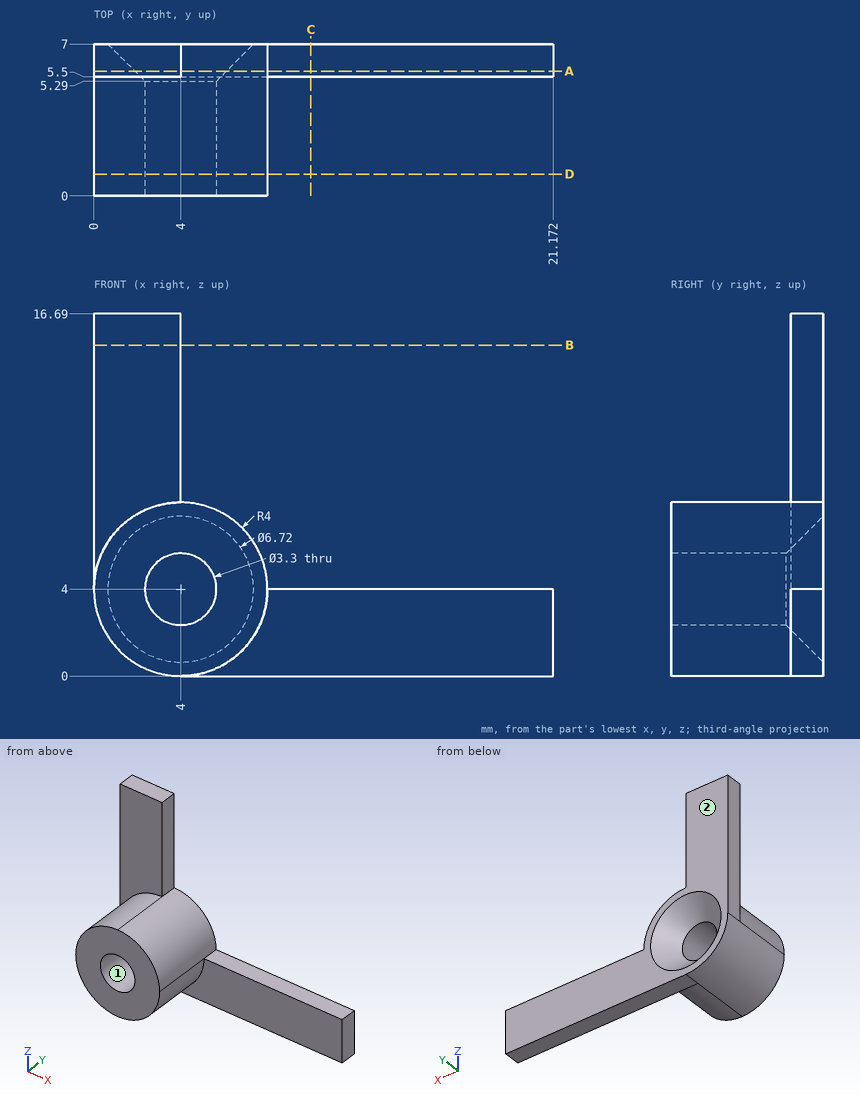
Source: three-view drawing plus pictorial views. Frame: mm from the lowest corner of the part. Coordinates: 2 decimals unless noted, no trailing zeros. Order: outer loops, then holes, each group sorted by start corner. A loop starts at its lowest first (then second) coordinate and runs counter-clockwise, first axis right, second up. Notation, with made-up numbers: M -32.5,35 L -15.5,35 A30 ccw -15.5,68 Z; hole C 26.5,57.5 d4. An arc over 180 degrees is marked long. Answer in a Markdown table with one row per item.
(1) Section query A-A, the plane y = 5.75. Output: boundary loops of the cut face in (x, z), plus the area to 3 significant figures.
Numbers:
| item | result |
|---|---|
| outline | M 0,4 A4 ccw 4,0 L 21.17,0 L 21.17,4 L 8,4 A4 ccw 4,8 L 4,16.69 L 0,16.69 Z; hole C 4,4 d4.22 |
| area | 131 mm^2 |
(2) Section query D-D, the plane y = 1. Output: boundary loops of the cut face in (x, z).
Numbers:
| item | result |
|---|---|
| outline | C 4,4 d8; hole C 4,4 d3.3 |
(3) Section query B-B, the plane z = 15.25. Output: boundary loops of the cut face in (x, y).
Numbers:
| item | result |
|---|---|
| outline | M 0,5.5 L 4,5.5 L 4,7 L 0,7 Z |
(4) Contact query for flat-ended pins moving along their axis: pin 1 Ø5.5 at (x, z) = (4, 4) entering from +Y; pin 2 Ø1.6 at (x, y) = (13.5, 6.5) entering from +Z; pin 3 Ø2 at (x, z) = (10.5, 2.5) entering from -Y. Output: stop coordinate, or through.
Numbers:
| item | result |
|---|---|
| pin 1 | stops at y = 6.39 |
| pin 2 | stops at z = 4 |
| pin 3 | stops at y = 5.5 |
(5) Material intervals for line 1 (X direction, y = 1.95, z = 4); line 2 (X direction, y = 6.75, z = 4.5), sorted ascending. Write a range as [from, to].
Numbers:
| item | result |
|---|---|
| line 1 | x = [0, 2.35], [5.65, 8] |
| line 2 | x = [0, 0.93], [7.07, 7.97] |
(6) Section query C-C, the plane x = 10. Output: boundary loops of the cut face in (y, z).
Numbers:
| item | result |
|---|---|
| outline | M 5.5,0 L 7,0 L 7,4 L 5.5,4 Z |
(7) Draft query along Z for the marked faces 1 and 2. Return one class per face: pulls with the +Z half, pulls with the -Z half, needs draft (parallel to the pull), parting line crosses it, or undercut.
Numbers:
| item | result |
|---|---|
| face 1 | undercut |
| face 2 | needs draft |
